```python
from build123d import *

# Parameters (mm, degrees)
SKETCH_1_W                     = 50
SKETCH_1_H                     = 100
EXTRUDE_1_DEPTH                = 2
SKETCH_2_W                     = 3
SKETCH_2_H                     = 100
EXTRUDE_2_DEPTH                = 80
SKETCH_3_W                     = 2
SKETCH_3_H                     = 66.7
EXTRUDE_3_DEPTH                = 70
CUT_EXTRUDE_4_REACH            = 162.465
SKETCH_8_W                     = 2
SKETCH_8_H                     = 66.7
EXTRUDE_4_DEPTH                = 70
CUT_EXTRUDE_5_REACH            = 140.25
HOLE_WIZARD_M3_1_D             = 2.5
HOLE_WIZARD_M3_1_DEPTH         = 2
HOLE_WIZARD_M3_1_CSINK_D       = 3.05
HOLE_WIZARD_M3_1_CSINK_ANGLE   = 90
FILLET_1_R                     = 2
CUT_EXTRUDE_6_REACH            = 140.25
SKETCH_12_R                    = 11
CUT_EXTRUDE_7_REACH            = 162.465
SKETCH_13_R                    = 14.5
SKETCH_14_W                    = 2
SKETCH_14_H                    = 66.7
EXTRUDE_5_DEPTH                = 70
CUT_EXTRUDE_8_REACH            = 156.14
SKETCH_15_R                    = 5.1
CUT_EXTRUDE_9_DEPTH            = 155.140358116
CUT_EXTRUDE_9_DEPTH_BACK       = 155.140358116
SKETCH_19_W                    = 2
SKETCH_19_H                    = 66.7
CUT_EXTRUDE_10_DEPTH           = 119.844436134
FILLET_2_R                     = 2
CUT_EXTRUDE_11_DEPTH           = 134.88427839
CUT_EXTRUDE_11_DEPTH_BACK      = 134.88427839
HOLE_WIZARD_M2_5_1_D           = 2.05
HOLE_WIZARD_M2_5_1_CSINK_D     = 2.55
HOLE_WIZARD_M2_5_1_CSINK_ANGLE = 90


with BuildPart() as part:
    # 草图1 → 凸台-拉伸1 (new body)
    with BuildSketch(Plane(origin=(0, 0, 0), x_dir=(1, 0, 0), z_dir=(0, 1, 0))):
        Rectangle(SKETCH_1_W, SKETCH_1_H)
    extrude(amount=EXTRUDE_1_DEPTH)

    # 草图2 → 凸台-拉伸2 (add)
    with BuildSketch(Plane(origin=(0, 2, 0), x_dir=(1, 0, 0), z_dir=(0, 1, 0))):
        with Locations((-23.5, 0)):
            Rectangle(SKETCH_2_W, SKETCH_2_H)
    extrude(amount=EXTRUDE_2_DEPTH)

    # 草图3 → 凸台-拉伸3 (add)
    with BuildSketch(Plane.ZY.offset(25)):
        with Locations((-49, 48.65)):
            Rectangle(SKETCH_3_W, SKETCH_3_H)
    extrude(amount=EXTRUDE_3_DEPTH)

    # 草图4 → 切除-拉伸4 (cut, up to next)
    with BuildSketch(Plane(origin=(0, 0, -50), x_dir=(-1, 0, 0), z_dir=(0, 0, -1)), mode=Mode.PRIVATE) as cut_extrude_4_sk1:
        with BuildLine():
            Line((95, 82), (61.65, 82))
            ThreePointArc((61.65, 82), (85.232011153, 72.232011153), (95, 48.65))
            Line((95, 48.65), (95, 82))
        make_face()
    cut_extrude_4_tool1 = extrude(cut_extrude_4_sk1.sketch, amount=-CUT_EXTRUDE_4_REACH, mode=Mode.PRIVATE) & part.part
    # 草图4 → 切除-拉伸4 (cut, up to next)
    with BuildSketch(Plane(origin=(0, 0, -50), x_dir=(-1, 0, 0), z_dir=(0, 0, -1)), mode=Mode.PRIVATE) as cut_extrude_4_sk2:
        with BuildLine():
            ThreePointArc((95, 48.65), (85.232011153, 25.067988847), (61.65, 15.3))
            Line((61.65, 15.3), (95, 15.3))
            Line((95, 15.3), (95, 48.65))
        make_face()
    cut_extrude_4_tool2 = extrude(cut_extrude_4_sk2.sketch, amount=-CUT_EXTRUDE_4_REACH, mode=Mode.PRIVATE) & part.part
    add(cut_extrude_4_tool1.solids().sort_by_distance((-87.550679, 74.550679, -50))[0], mode=Mode.SUBTRACT)
    add(cut_extrude_4_tool2.solids().sort_by_distance((-87.550679, 22.749321, -50))[0], mode=Mode.SUBTRACT)

    # 草图8 → 凸台-拉伸4 (add)
    with BuildSketch(Plane.ZY.offset(25)):
        with Locations((7, 48.65)):
            Rectangle(SKETCH_8_W, SKETCH_8_H)
    extrude(amount=EXTRUDE_4_DEPTH)

    # 草图9 → 切除-拉伸5 (cut, up to next)
    with BuildSketch(Plane.XY.offset(8), mode=Mode.PRIVATE) as cut_extrude_5_sk1:
        with BuildLine():
            ThreePointArc((-95, 48.65), (-85.232011153, 72.232011153), (-61.65, 82))
            Line((-61.65, 82), (-95, 82))
            Line((-95, 82), (-95, 48.65))
        make_face()
    cut_extrude_5_tool1 = extrude(cut_extrude_5_sk1.sketch, amount=-CUT_EXTRUDE_5_REACH, mode=Mode.PRIVATE) & part.part
    # 草图9 → 切除-拉伸5 (cut, up to next)
    with BuildSketch(Plane.XY.offset(8), mode=Mode.PRIVATE) as cut_extrude_5_sk2:
        with BuildLine():
            ThreePointArc((-61.65, 15.3), (-85.232011153, 25.067988847), (-95, 48.65))
            Line((-95, 48.65), (-95, 15.3))
            Line((-95, 15.3), (-61.65, 15.3))
        make_face()
    cut_extrude_5_tool2 = extrude(cut_extrude_5_sk2.sketch, amount=-CUT_EXTRUDE_5_REACH, mode=Mode.PRIVATE) & part.part
    add(cut_extrude_5_tool1.solids().sort_by_distance((-87.550679, 74.550679, 8))[0], mode=Mode.SUBTRACT)
    add(cut_extrude_5_tool2.solids().sort_by_distance((-87.550679, 22.749321, 8))[0], mode=Mode.SUBTRACT)

    # M3 螺纹孔1
    with Locations(Plane.XY.offset(8)):
        with Locations((-78.970508076, 38.65), (-61.65, 68.65), (-44.329491924, 38.65)):
            CounterSinkHole(HOLE_WIZARD_M3_1_D / 2, HOLE_WIZARD_M3_1_CSINK_D / 2, depth=HOLE_WIZARD_M3_1_DEPTH, counter_sink_angle=HOLE_WIZARD_M3_1_CSINK_ANGLE)

    # 圆角1
    fillet_1_edges = [part.edges().sort_by_distance(p)[0] for p in [
        (-23.5, 82, 50),
        (25, 1, 50),
        (25, 1, -50),
    ]]
    fillet(fillet_1_edges, radius=FILLET_1_R)

    # 草图12 → 切除-拉伸6 (cut, up to next)
    with BuildSketch(Plane.XY.offset(8), mode=Mode.PRIVATE) as cut_extrude_6_sk1:
        with Locations((-61.65, 48.65)):
            Circle(SKETCH_12_R)
    cut_extrude_6_tool1 = extrude(cut_extrude_6_sk1.sketch, amount=-CUT_EXTRUDE_6_REACH, mode=Mode.PRIVATE) & part.part
    add(cut_extrude_6_tool1.solids().sort_by_distance((-61.65, 48.65, 8))[0], mode=Mode.SUBTRACT)

    # 草图13 → 切除-拉伸7 (cut, up to next)
    with BuildSketch(Plane(origin=(0, 0, -50), x_dir=(-1, 0, 0), z_dir=(0, 0, -1)), mode=Mode.PRIVATE) as cut_extrude_7_sk1:
        with Locations((61.65, 48.65)):
            Circle(SKETCH_13_R)
    cut_extrude_7_tool1 = extrude(cut_extrude_7_sk1.sketch, amount=-CUT_EXTRUDE_7_REACH, mode=Mode.PRIVATE) & part.part
    add(cut_extrude_7_tool1.solids().sort_by_distance((-61.65, 48.65, -50))[0], mode=Mode.SUBTRACT)

    # 草图14 → 凸台-拉伸5 (add)
    with BuildSketch(Plane.ZY.offset(25)):
        with Locations((-38.5, 48.65)):
            Rectangle(SKETCH_14_W, SKETCH_14_H)
    extrude(amount=EXTRUDE_5_DEPTH)

    # 草图15 → 切除-拉伸8 (cut, up to next)
    with BuildSketch(Plane(origin=(0, 0, -39.5), x_dir=(-1, 0, 0), z_dir=(0, 0, -1)), mode=Mode.PRIVATE) as cut_extrude_8_sk1:
        with Locations(Location((61.65, 48.65, 0), (0, 0, 90))):
            Circle(SKETCH_15_R)
    cut_extrude_8_tool1 = extrude(cut_extrude_8_sk1.sketch, amount=-CUT_EXTRUDE_8_REACH, mode=Mode.PRIVATE) & part.part
    add(cut_extrude_8_tool1.solids().sort_by_distance((-61.65, 48.65, -39.5))[0], mode=Mode.SUBTRACT)

    # 草图18 → 切除-拉伸9 (cut, two sides: drawn at the far end of the back side and taken through both)
    with BuildSketch(Plane(origin=(0, 0, -39.5), x_dir=(-1, 0, 0), z_dir=(0, 0, -1)).offset(-CUT_EXTRUDE_9_DEPTH_BACK)):
        with BuildLine():
            Line((95, 15.3), (95, 48.65))
            ThreePointArc((95, 48.65), (85.232011153, 25.067988847), (61.65, 15.3))
            Line((61.65, 15.3), (95, 15.3))
        make_face()
        with BuildLine():
            Line((95, 48.65), (95, 82))
            Line((95, 82), (61.65, 82))
            ThreePointArc((61.65, 82), (85.232011153, 72.232011153), (95, 48.65))
        make_face()
    extrude(amount=CUT_EXTRUDE_9_DEPTH + CUT_EXTRUDE_9_DEPTH_BACK, mode=Mode.SUBTRACT)

    # 草图19 → 切除-拉伸10 (cut, through all)
    with BuildSketch(Plane.ZY.offset(25)):
        with Locations((-49, 48.65)):
            Rectangle(SKETCH_19_W, SKETCH_19_H)
    extrude(amount=CUT_EXTRUDE_10_DEPTH, mode=Mode.SUBTRACT)

    # 圆角2
    fillet_2_edges = [part.edges().sort_by_distance(p)[0] for p in [
        (-23.5, 82, -50),
    ]]
    fillet(fillet_2_edges, radius=FILLET_2_R)

    # 草图20 → 切除-拉伸11 (cut, two sides: drawn at the far end of the back side and taken through both)
    with BuildSketch(Plane(origin=(0, 2, 0), x_dir=(1, 0, 0), z_dir=(0, 1, 0)).offset(-CUT_EXTRUDE_11_DEPTH_BACK)):
        Polygon((-25, -8), (-95, -8), (-95, -6), (-25, -6), (-25, 50), (25, 50), (25, -50), (-25, -50), align=None)
    extrude(amount=CUT_EXTRUDE_11_DEPTH + CUT_EXTRUDE_11_DEPTH_BACK, mode=Mode.SUBTRACT)

    # M2.5 螺纹孔1 (through all)
    with Locations(Plane.XY.offset(-37.5)):
        with Locations((-29, 52.65), (-29, 44.65)):
            CounterSinkHole(HOLE_WIZARD_M2_5_1_D / 2, HOLE_WIZARD_M2_5_1_CSINK_D / 2, counter_sink_angle=HOLE_WIZARD_M2_5_1_CSINK_ANGLE)


solid = part.part
```
Design review of the part built by this model. Coordinates are the model's own, in mm. Coordinates: 2 decimals unless noted, no trailing zeros. Loops run counter-clockwise (first coordinate to the right, second up) from the corner with the lowest first, then second, coordinate; pieces in that order, holes last. Notation, with made-up numbers: (37.25, 54.5) -> (43.25, 54.5) arc R21 ccw to (43.25, 69.5) -> close; hole circle Ø8 at (33.25, 61). An arc over 180 degrees is marked (long way). Answer as a JSON object with one key per item and string values.
Q1. Take a section at B-B on z = -38.15. Give the boundary of the cut face in (x, y) (3 decimals), plus the area to 3 significant figures.
Answer block:
{"outline": "(-61.65, 15.3) -> (-25, 15.3) -> (-25, 82) -> (-61.65, 82) arc R33.35 ccw to start; hole circle Ø10.2 at (-61.65, 48.65); hole circle Ø2.05 at (-29, 44.65); hole circle Ø2.05 at (-29, 52.65)", "area": "4,100 mm^2"}
Q2. Take a section at C-C on y = 52.65. Give the boundary of the cut face in (x, z) (3 decimals).
Answer block:
{"outline": "(-94.759, -39.5) -> (-64.814, -39.5) -> (-64.814, -37.5) -> (-94.759, -37.5) -> close; (-58.486, -39.5) -> (-30.025, -39.5) -> (-30.025, -37.75) -> (-30.275, -37.5) -> (-58.486, -37.5) -> close; (-27.975, -39.5) -> (-25, -39.5) -> (-25, -37.5) -> (-27.725, -37.5) -> (-27.975, -37.75) -> close"}
Q3. Clearance check with flat-ended pins moving along their axes: pin 1 Ø1.8 at (x, y) = (-29, 44.65) entering from +Z; pin 2 Ø1 at (x, z) = (-75.5, -38.5) entering from -Y. State where each tip first meets the part, or that it passes through.
Answer block:
{"pin 1": "passes through", "pin 2": "stops at y = 18.09"}
Q4. Take a section at A-A on x = -29. Give the boundary of the cut face in (y, z) (3 decimals).
Answer block:
{"outline": "(15.3, -39.5) -> (43.625, -39.5) -> (43.625, -37.75) -> (43.375, -37.5) -> (15.3, -37.5) -> close; (45.675, -39.5) -> (51.625, -39.5) -> (51.625, -37.75) -> (51.375, -37.5) -> (45.925, -37.5) -> (45.675, -37.75) -> close; (53.675, -39.5) -> (82, -39.5) -> (82, -37.5) -> (53.925, -37.5) -> (53.675, -37.75) -> close"}
Q5. To check wall thickness, follow L1, parallel to Y at x = -29, z = -38.2 (3 decimals); L2, parallel to X at y = 48.65, z = -38; L3, parallel to X at y = 45.5, z = -38.75. State the ranges of each line that lie inside material, in increasing order.
Answer block:
{"L1": "y = 15.3 to 43.625, 45.675 to 51.625, 53.675 to 82", "L2": "x = -95 to -66.75, -56.55 to -25", "L3": "x = -94.85 to -65.66, -57.64 to -29.57, -28.43 to -25"}
Q6. Take a section at D-D on y = 74.5. Give the boundary of the cut face in (x, z).
Answer block:
{"outline": "(-82.72, -39.5) -> (-25, -39.5) -> (-25, -37.5) -> (-82.72, -37.5) -> close"}
Q7. The part is to be moulded in two halves that separate along X. For faces 1 (the cylindrical face through (-57.35, 51.39, -38.51)), 2 (the cylindrical face through (-28.867, 45.666, -38.637)), 3 (the flat face through (-25, 48, -38)), 4 (the flat face through (-43, 15.3, -39)), say which applies: +X half, -X half, draft (parallel to the pull), parting line (faces both ways), or undercut.
Answer block:
{"face 1": "undercut", "face 2": "undercut", "face 3": "+X half", "face 4": "draft"}
